Part model, mm, in its own coordinate system. Face numbers are marked on the shaded views. A direction names the side the tool comes from. Coordinates: 2 decimals unless noted, no trailing zeros. Write each loop counter-clockwise with the first axis right and the second up, starting at its lowest first coordinate (ties: lowest second). Pieces come first, ordered by that corner, then holes. Notation, with made-up numbers: (33.5, 52.5) -> (68.5, 52.5) arc R17 ccw to (68.5, 56.5) -> close; hole circle Ø11 at (2, 79.25). An arc over 180 degrees is marked (long way). One line per question, with ' | ' between items. Start each with the question number.
Item 1: Saw through at B-B (x = -24.5). List the corners of the cut face in (y, z) (3 decimals).
Item 2: Probe probe 1 along X at (y, z) = (-25, -14); probe 2 along Z at (x, y) = (-31.75, -27.5); probe 3 along X at (y, z) = (-31, -3). List the from-to ranges inside material, lowest first. Write a range as [from, to].
Item 3: 3-axis set-ups, long thin cutter, end or side, ignore diameter. For the marked faces 1, 2 and 3: which of +Z, -Z, +X, -X, +Y, -Y reach the whole face in a straight line?
Item 4: Pin check, flat tips, straight feed: pin 1 (5 mm diameter, centred on x = -20.5, z = -21, fed in from -Y); pin 2 (4.5 mm diameter, centred on y = -42, z = -45.5, fed in from +X); pin 3 (4 mm diameter, centred on x = -36.5, y = -7.5, fed in from -Z); pin 4 (10 mm diameter, centred on x = -25, y = -16.5, fed in from -Z). Stop position of each tip, or through.
Item 5: Saw through at A-A (y = -6). List the corners of the cut face in (x, z), and give its area (3 significant figures).
Item 6: Saw through at C-C (x = -37.75). List the corners of the cut face in (y, z), and give its area (3 significant figures).
Item 7: Two-plate mould, pull along X, no slides. Class the marked faces 4, 5 and 6: pulls with the +X half, pulls with the -X half, needs draft (parallel to the pull), parting line crosses it, or undercut.
Item 8: Saw through at D-D (z = -32.5). List the corners of the cut face in (x, y), and give its area (3 significant figures).
from build123d import *

# Parameters (mm, degrees)
SKETCH_W        = 28
SKETCH_H        = 42
PAD_DEPTH       = 48
POCKET_DEPTH    = 42.001
POCKET001_DEPTH = 28.001
POCKET002_DEPTH = 40
POCKET003_DEPTH = 42.001
SKETCH005_W     = 12.884712
SKETCH005_H     = 5
PAD001_DEPTH    = 10
SKETCH006_W     = 8
SKETCH006_H     = 5
PAD002_DEPTH    = 6
SKETCH007_W     = 9
SKETCH007_H     = 5
PAD003_DEPTH    = 13
SKETCH009_R     = 1.75
POCKET004_DEPTH = 6
SKETCH010_W     = 16.115288
SKETCH010_H     = 23
PAD004_DEPTH    = 1
SKETCH011_W     = 16.115288
SKETCH011_H     = 10.869565
PAD005_DEPTH    = 1


with BuildPart() as part:
    # Sketch → Pad (new body)
    with BuildSketch(Plane.XY):
        with Locations((-29, -29)):
            Rectangle(SKETCH_W, SKETCH_H)
    extrude(amount=-PAD_DEPTH)

    # Sketch001 (on Face3 of Pad) → Pocket (cut, through all)
    with BuildSketch(Plane.XZ.offset(50)):
        with BuildLine():
            ThreePointArc((-43, -17.83216), (-32.688295, -36.339337), (-15, -48))
            Line((-15, -48), (-62.101535, -92.662663))
            Line((-43, -17.83216), (-62.101535, -92.662663))
        make_face()
    extrude(amount=-POCKET_DEPTH, mode=Mode.SUBTRACT)

    # Sketch002 (on Face3 of Pocket) → Pocket001 (cut, through all)
    with BuildSketch(Plane.YZ.offset(-15)):
        Polygon((0, 10), (-23, -50), (20.241647, -57.218418), align=None)
    extrude(amount=-POCKET001_DEPTH, mode=Mode.SUBTRACT)

    # Sketch003 (on Face1 of Pocket001) → Pocket002 (cut)
    with BuildSketch(Plane(origin=(0, -8, 0), x_dir=(-1, 0, 0), z_dir=(0, 1, 0))):
        with BuildLine():
            Line((41.5, 3), (41.5, -17.25833))
            ThreePointArc((12.43, -47.164245), (30.833459, -35.971617), (41.5, -17.25833))
            Line((12.43, -44.72372), (12.43, -47.164245))
            ThreePointArc((12.43, -44.72372), (23.996206, -23.678239), (28, 0))
            Line((28, 3), (28, 0))
            Line((41.5, 3), (28, 3))
        make_face()
    extrude(amount=-POCKET002_DEPTH, mode=Mode.SUBTRACT)

    # Sketch004 (on Face10 of Pocket002) → Pocket003 (cut, through all)
    with BuildSketch(Plane.XZ.offset(50)):
        with BuildLine():
            ThreePointArc((-26, 0), (-13.012856, -42.489763), (21.51, -70.45793))
            Line((21.51, -70.45793), (50, 0))
            Line((-26, 0), (50, 0))
        make_face()
    extrude(amount=-POCKET003_DEPTH, mode=Mode.SUBTRACT)

    # Sketch005 (on Face1 of Pocket003) → Pad001 (join)
    with BuildSketch(Plane(origin=(0, -8, 0), x_dir=(-1, 0, 0), z_dir=(0, 1, 0))):
        with Locations((20.442356, -2.5)):
            Rectangle(SKETCH005_W, SKETCH005_H)
    extrude(amount=-PAD001_DEPTH)

    # Sketch006 (on Face13 of Pad001) → Pad002 (join)
    with BuildSketch(Plane(origin=(0, -8, 0), x_dir=(-1, 0, 0), z_dir=(0, 1, 0))):
        with Locations((18, -2.5)):
            Rectangle(SKETCH006_W, SKETCH006_H)
    extrude(amount=PAD002_DEPTH)

    # Sketch007 (on Face11 of Pad002) → Pad003 (join)
    with BuildSketch(Plane.XZ.offset(50)):
        with Locations((-22.5, -2.5)):
            Rectangle(SKETCH007_W, SKETCH007_H)
    extrude(amount=-PAD003_DEPTH)

    # Sketch009 (on Face24 of Pad003) → Pocket004 (cut)
    with BuildSketch(Plane.XY):
        with Locations((-18, -6)):
            Circle(SKETCH009_R)
        with Locations((-22, -40)):
            Circle(SKETCH009_R)
    extrude(amount=-POCKET004_DEPTH, mode=Mode.SUBTRACT)

    # Sketch010 (on Face2 of Pocket004) → Pad004 (join)
    with BuildSketch(Plane.XY):
        with Locations((-34.942356, -38.5)):
            Rectangle(SKETCH010_W, SKETCH010_H)
    extrude(amount=-PAD004_DEPTH)

    # Sketch011 (on Face39 of Pad004) → Pad005 (join)
    with BuildSketch(Plane(origin=(0, -8, 0), x_dir=(-1, 0, 0), z_dir=(0, 1, 0))):
        with Locations((34.942356, -5.434782)):
            Rectangle(SKETCH011_W, SKETCH011_H)
    extrude(amount=-PAD005_DEPTH)


solid = part.part
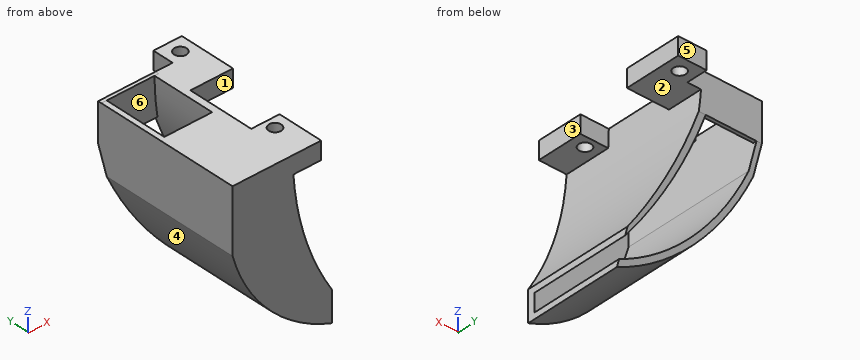
From the geometry:
1) outline: (-50, -43.266) -> (-20.419, -43.266) -> (-19.679, -41.338) -> (-48, -41.338) -> (-48, -22.178) -> (-12.335, -22.178) -> (-9.593, -15.025) -> (-50, -15.025) -> close; (-50, -5) -> (-37, -5) -> (-37, 0) -> (-50, 0) -> close; (-18, -5) -> (-8, -5) -> (-8, 0) -> (-18, 0) -> close
2) probe 1: [-43, -41.5], [-26.63, -24.7] | probe 2: [-37.32, -35], [-1, 0] | probe 3: [-43, -41.5], [-27.94, -25.94]
3) face 1: +Z, +X | face 2: +X, +Y, -Y | face 3: +Z, +X, -Y
4) pin 1: y = -50 | pin 2: x = -15 | pin 3: z = -10.87 | pin 4: z = -44.46
5) outline: (-22, -5) -> (-19.75, -5) -> (-19.75, 0) -> (-22, 0) -> close; (-16.25, -5) -> (-14, -5) -> (-14, 0) -> (-16.25, 0) -> close | area: 22.5 mm2
6) outline: (-50, -29.75) -> (-15.24, -29.75) -> (-14.03, -26.59) -> (-48, -26.59) -> (-48, -1) -> (-27, -1) -> (-27, 0) -> (-50, 0) -> close; (-9, -10.87) -> (-8, -10.87) -> (-8, 0) -> (-9, 0) -> close | area: 197 mm2
7) face 4: pulls with the -X half | face 5: needs draft | face 6: undercut
8) outline: (-35.87, -50) -> (-18.7, -50) -> (-18.7, -16.29) -> (-20.25, -16.29) -> (-20.25, -48) -> (-33.86, -48) -> (-33.86, -16.29) -> (-35.87, -16.29) -> close | area: 147 mm2
